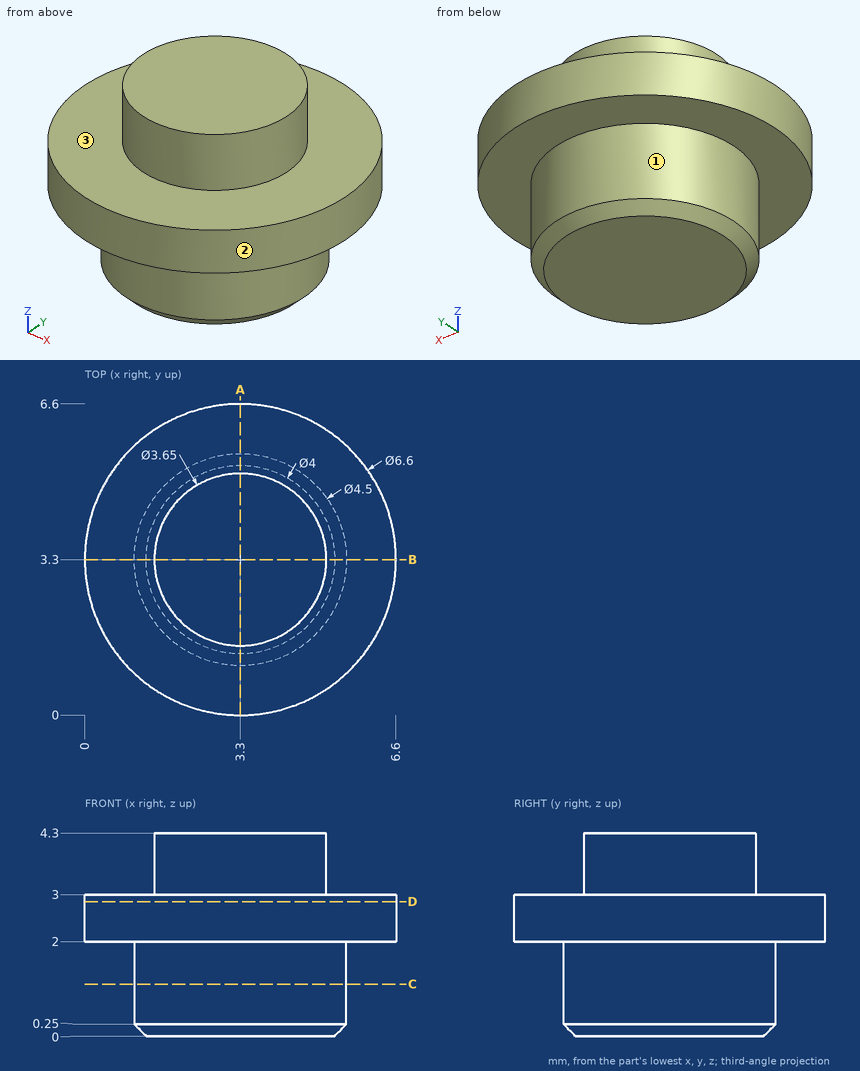
The drawing under review shows one solid part. Ordinate dimensions are in mm from its lowest x, y, z. A direction names the side the tool comes from. Coordinates: 2 decimals unless noted, no trailing zeros. Write each loop counter-clockwise with the first axis right and the second up, starting at its lowest first coordinate (ties: lowest second). Pieces come first, ordered by that corner, then holes. Notation, with made-up numbers: (45, 63) -> (61, 63) arc R17 cw to (61, 69) -> close; hole circle Ø1 at (-18.75, -25.5). An arc over 180 degrees is marked (long way). One line per item, written item: value. Start each with the question number.
Q1. Add section A-A, the plane x = 3.3. Give the boundary of the cut face in (y, z) (3 decimals).
Q2. Add section C-C, the plane z = 1.1. Give the boundary of the cut face in (x, y).
Q3. Clearance check with flat-ended pins moving along their axes: P1, Ø2, axis at x = 2, y = 1.5, coming from the +Z side; P2, Ø1, axis at y = 3, z = 0.5, coming from the +X side; P3, Ø1.5, axis at x = 6, y = 1.5, coming from the -Z side. State where each tip first meets the part, or that it passes through.
Q4. Add section D-D, the plane z = 2.85. Give the boundary of the cut face in (x, y), then the cut area to 3 significant figures.
Q5. To check wall thickness, follow probe 1 along Z at (x, y) = (6.5, 3); probe 2 along Z at (x, y) = (2.25, 1.75); probe 3 along X at (y, z) = (3.25, 3.65). State the ranges of each line that lie inside material, in increasing order.
Q6. For the marked faces 1, 2 and 3, list the 3-axis set-ups (+Z, -Z, +X, -X, +Y, -Y) from which the entire face can be reached by the end or side of a thin tool; tool diameter is ignored.
Response:
1. outline: (0, 2) -> (1.05, 2) -> (1.05, 0.25) -> (1.3, 0) -> (5.3, 0) -> (5.55, 0.25) -> (5.55, 2) -> (6.6, 2) -> (6.6, 3) -> (5.125, 3) -> (5.125, 4.3) -> (1.475, 4.3) -> (1.475, 3) -> (0, 3) -> close
2. outline: circle Ø4.5 at (3.3, 3.3)
3. P1: z = 4.3
3. P2: x = 5.55
3. P3: z = 2
4. outline: circle Ø6.6 at (3.3, 3.3)
4. area: 34.2 mm²
5. probe 1: 2 to 3
5. probe 2: 0 to 3
5. probe 3: 1.48 to 5.12
6. face 1: -Z
6. face 2: +Z, -Z
6. face 3: +Z
